Verification items for this drawing (mm, ordinates from the low corner). Give positions to 0.01 mm unless a question says otherwise; leave off trailing zeros. Loops run counter-clockwise (first coordinate to the right, second up) from the corner with the lowest first, then second, coordinate; pieces in that order, holes last. Notation, with made-up numbers: (66.5, 72.25) -> (82.5, 72.25) arc R11 cw to (82.5, 78.25) -> close; hole circle Ø11 at (62, -23). An arc over 180 degrees is marked (long way). Write each question's results on one line, items separated by ' | '. Start each with the question number.
Item 1: Gauge pin test, flat end, axial feed: pin 1 Ø2.5 at (x, z) = (24, 3) entering from +Y. Record the tip position at first contact, or that the pin passes through.
Item 2: Scan lines: line 1 along Z through (x, y) = (3, 1); line 2 along X through (y, z) = (1.4, 3); line 3 along Z through (x, y) = (2.25, 1.85). Record each from-to range of solid material in increasing order.
Item 3: Cross-section at B-B on x = 24.25. Enter the section's corners in (y, z), then the cut area to 3 significant figures.
Item 4: Cross-section at A-A on z = 58. Enter the section's corners in (x, y).
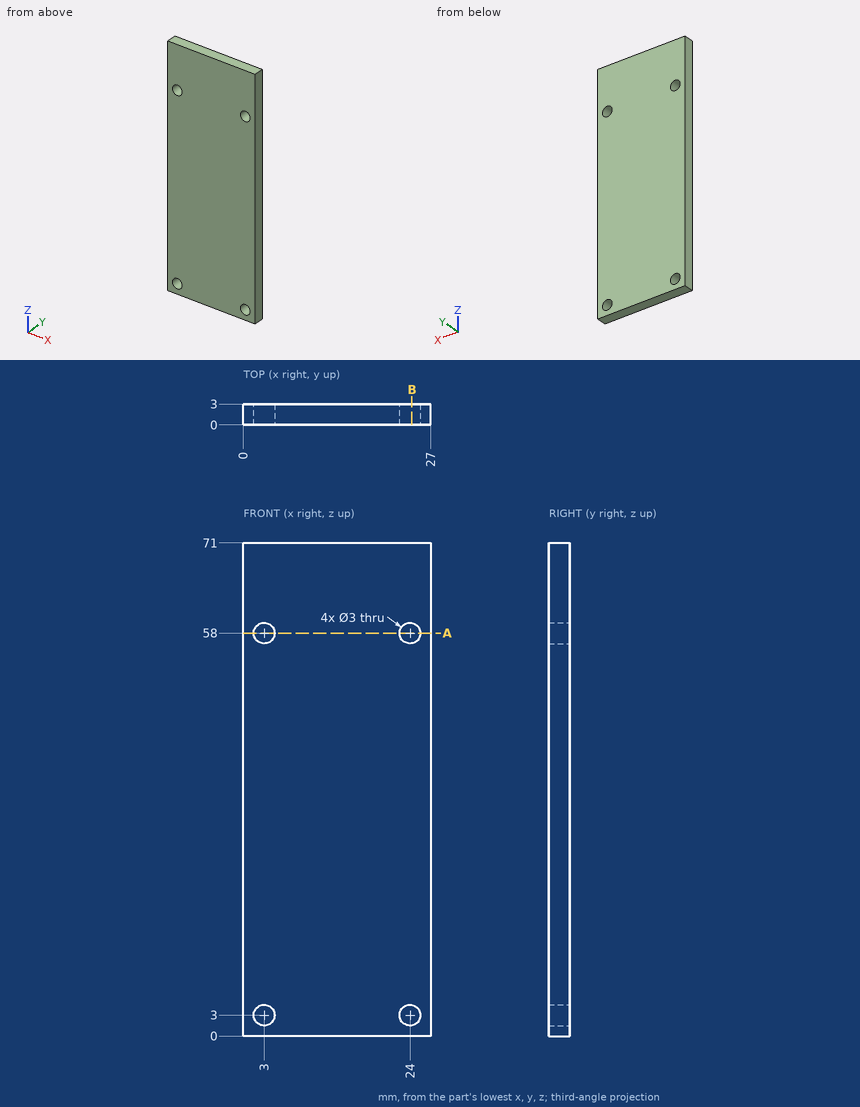
Answer sheet:
1) pin 1: passes through
2) line 1: z = 0 to 1.5, 4.5 to 56.5, 59.5 to 71 | line 2: x = 0 to 1.5, 4.5 to 22.5, 25.5 to 27 | line 3: z = 0 to 1.7, 4.3 to 56.7, 59.3 to 71
3) outline: (0, 0) -> (3, 0) -> (3, 1.52) -> (0, 1.52) -> close; (0, 4.48) -> (3, 4.48) -> (3, 56.52) -> (0, 56.52) -> close; (0, 59.48) -> (3, 59.48) -> (3, 71) -> (0, 71) -> close | area: 195 mm²
4) outline: (0, 0) -> (1.5, 0) -> (1.5, 3) -> (0, 3) -> close; (4.5, 0) -> (22.5, 0) -> (22.5, 3) -> (4.5, 3) -> close; (25.5, 0) -> (27, 0) -> (27, 3) -> (25.5, 3) -> close
